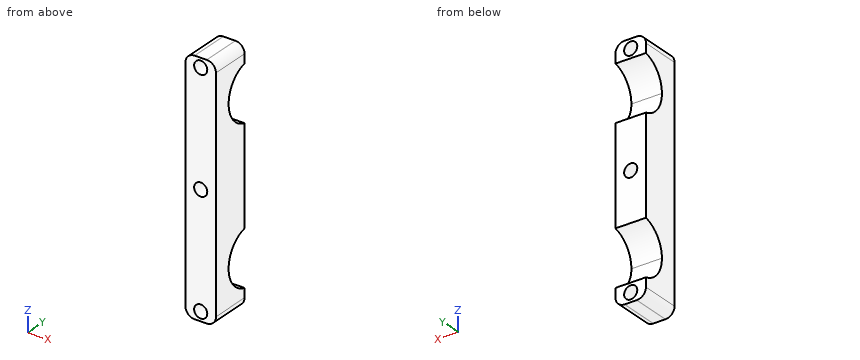
```python
from build123d import *

# Parameters (mm, degrees)
F0_R     = 2.15
F1_DEPTH = 13
F3_DEPTH = 25


# Not quite as in the source:
# - a feature names something its author has since deleted; it is built from what else it names


with BuildPart() as f1:
    # F0 (on Front) → F1 (new body)
    with BuildSketch(Plane.XZ):
        with BuildLine():
            Line((2, 38.987471127), (-2, 38.987471127))
            ThreePointArc((-2, 38.987471127), (-4.1213203436, 38.1087914705), (-5, 35.987471127))
            Line((-5, 35.987471127), (-5, -38.012528873))
            ThreePointArc((-5, -38.012528873), (-4.1213203436, -40.1338492166), (-2, -41.012528873))
            Line((-2, -41.012528873), (2, -41.012528873))
            ThreePointArc((2, -41.012528873), (4.1213203436, -40.1338492166), (5, -38.012528873))
            Line((5, -38.012528873), (5, 35.987471127))
            ThreePointArc((5, 35.987471127), (4.1213203436, 38.1087914705), (2, 38.987471127))
        make_face()
        with Locations((0, -38.012528873)):
            Circle(F0_R, mode=Mode.SUBTRACT)
        with Locations((0, -1.012528873)):
            Circle(F0_R, mode=Mode.SUBTRACT)
        with Locations((0, 35.987471127)):
            Circle(F0_R, mode=Mode.SUBTRACT)
    extrude(amount=F1_DEPTH)

    # F2 (on face) → F3 (cut)
    with BuildSketch(Plane(origin=(-5, 0, 0), x_dir=(0, -1, 0), z_dir=(-1, 0, 0))):
        with BuildLine():
            ThreePointArc((0, 14.9562751929), (5.2132690231, 18.196853716), (7.25, 23.987471127))
            ThreePointArc((7.25, 23.987471127), (5.2132690231, 29.7780885379), (0, 33.0186670611))
            Line((0, 33.0186670611), (0, 23.987471127))
            Line((0, 23.987471127), (0, 14.9562751929))
        make_face()
        with BuildLine():
            ThreePointArc((7.25, -26.012528873), (5.2132690231, -20.2219114621), (0, -16.9813329389))
            Line((0, -16.9813329389), (0, -35.0437248071))
            ThreePointArc((0, -35.0437248071), (5.2132690231, -31.803146284), (7.25, -26.012528873))
        make_face()
    extrude(amount=-F3_DEPTH, mode=Mode.SUBTRACT)


solid = f1.part
```
CAD build for the part. Positions are in the model's coordinates, mm. Coordinates: 2 decimals unless noted, no trailing zeros. Order: outer loops, then holes, each group sorted by start corner. A loop starts at its lowest first (then second) coordinate and runs counter-clockwise, first axis right, second up. Notation, with made-up numbers: (-9, 61.25) -> (34, 61.25) arc R18 ccw to (34, 71.25) -> close; hole circle Ø5 at (12, 6.25). An arc over 180 degrees is marked (long way). Use one line per item in the form item = value. Start each with the question number.
1) Band-saw the part on B-B on x = 0. Give the cut face in (y, z).
2) Drill centre lines: L1, parallel to Z at x = 0, y = -8.5; L2, parallel to Z at x = 1.75, y = -5; L3, parallel to Z at x = -3.5, y = -1. Where is each one in solid material? Low to high. Write a range as [from, to].
3) Band-saw the part on D-D on x = 3. Give the cut face in (y, z), then the cut area to 3 significant figures.
4) Drop flat-ended pins along their axis: pin 1 (4 mm diameter, centred on x = 0, z = -1.01, fed in from +Y); pin 2 (4 mm diameter, centred on x = 3.5, y = -9, fed in from -Z). Give the stop position or say it passes through.
5) Band-saw the part on A-A on y = -0.75. Give the cut face in (x, z), then the cut area to 3 significant figures.
6) Band-saw the part on C-C on y = -6.25. Give the cut face in (x, z).
Entries:
q1.outline = (-13, -41.01) -> (0, -41.01) -> (0, -40.16) -> (-13, -40.16) -> close; (-13, -35.86) -> (0, -35.86) -> (0, -35.04) arc R9.25 cw to (0, -16.98) -> (0, -3.16) -> (-13, -3.16) -> close; (-13, 1.14) -> (0, 1.14) -> (0, 14.96) arc R9.25 cw to (0, 33.02) -> (0, 33.84) -> (-13, 33.84) -> close; (-13, 38.14) -> (0, 38.14) -> (0, 38.99) -> (-13, 38.99) -> close
q2.L1 = [-41.01, -40.16], [-35.86, -3.16], [1.14, 33.84], [38.14, 38.99]
q2.L2 = [-41.01, -39.26], [-36.76, -32.06], [-19.97, -2.26], [0.24, 17.94], [30.03, 34.74], [37.24, 38.99]
q2.L3 = [-40.61, -34.76], [-17.26, 15.24], [32.74, 38.59]
q3.outline = (-13, -40.84) -> (0, -40.84) -> (0, -35.04) arc R9.25 cw to (0, -16.98) -> (0, 14.96) arc R9.25 cw to (0, 33.02) -> (0, 38.82) -> (-13, 38.82) -> close
q3.area = 840 mm2
q4.pin_1 = through
q4.pin_2 = -41.01
q5.outline = (-5, -38.01) arc R3 ccw to (-2, -41.01) -> (2, -41.01) arc R3 ccw to (5, -38.01) -> (5, -34.84) -> (-5, -34.84) -> close; (-5, -17.18) -> (5, -17.18) -> (5, 15.16) -> (-5, 15.16) -> close; (-5, 32.82) -> (5, 32.82) -> (5, 35.99) arc R3 ccw to (2, 38.99) -> (-2, 38.99) arc R3 ccw to (-5, 35.99) -> close; hole circle Ø4.3 at (0, -38.01); hole circle Ø4.3 at (0, -1.01); hole circle Ø4.3 at (0, 35.99)
q5.area = 395 mm2
q6.outline = (-5, -38.01) arc R3 ccw to (-2, -41.01) -> (2, -41.01) arc R3 ccw to (5, -38.01) -> (5, -30.2) -> (-5, -30.2) -> close; (-5, -21.83) -> (5, -21.83) -> (5, 19.8) -> (-5, 19.8) -> close; (-5, 28.17) -> (5, 28.17) -> (5, 35.99) arc R3 ccw to (2, 38.99) -> (-2, 38.99) arc R3 ccw to (-5, 35.99) -> close; hole circle Ø4.3 at (0, -38.01); hole circle Ø4.3 at (0, -1.01); hole circle Ø4.3 at (0, 35.99)
